```python
from build123d import *

# Parameters (mm, degrees)
F0_W     = 5
F0_H     = 3
F0_W_2   = 14
F3_SIZE  = 0.5
F4_D     = 4.4
F4_DEPTH = 14
F4_TIP   = 1.3218933619
F5_SIZE  = 0.5
F7_D     = 4.4
F7_DEPTH = 14
F7_TIP   = 1.3218933619
F8_W     = 10
F8_H     = 1.5
F9_DEPTH = 10


with BuildPart() as f1:
    # F0 (on Front) → F1 (revolve)
    with BuildSketch(Plane.XZ):
        Polygon((-30.4, 3), (-30.4, 0), (30.4, 0), (30.4, 3), (30.4, 4), (5, 4), (-5, 4), (-30.4, 4), align=None)
        with Locations((-32.9, 1.5)):
            Rectangle(F0_W, F0_H)
        with Locations((37.4, 1.5)):
            Rectangle(F0_W_2, F0_H)
    revolve(axis=Axis((7.3750944167, 0, 0), (1, 0, 0)))

    # F3
    f3_edges = [f1.edges().sort_by_distance(p)[0] for p in [
        (44.4, 0, -3),
    ]]
    chamfer(f3_edges, length=F3_SIZE)

    # F4
    with Locations(Plane.YZ.offset(44.4)):
        with Locations((0, 0)):
            Hole(F4_D / 2, depth=F4_DEPTH)
            with Locations((0, 0, -(F4_DEPTH + F4_TIP / 2))):  # 118° drill point
                Cone(0, F4_D / 2, F4_TIP, mode=Mode.SUBTRACT)

    # F5
    f5_edges = [f1.edges().sort_by_distance(p)[0] for p in [
        (-35.4, 0, -3),
    ]]
    chamfer(f5_edges, length=F5_SIZE)

    # F7
    with Locations(Plane(origin=(-35.4, 0, 0), x_dir=(0, -1, 0), z_dir=(-1, 0, 0))):
        with Locations((0, 0)):
            Hole(F7_D / 2, depth=F7_DEPTH)
            with Locations((0, 0, -(F7_DEPTH + F7_TIP / 2))):  # 118° drill point
                Cone(0, F7_D / 2, F7_TIP, mode=Mode.SUBTRACT)

    # F8 (on Front) → F9 (cut, symmetric)
    with BuildSketch(Plane.XZ):
        with Locations((0.4, -3.25)):
            Rectangle(F8_W, F8_H)
        with Locations((0.4, 3.25)):
            Rectangle(F8_W, F8_H)
    extrude(amount=F9_DEPTH, both=True, mode=Mode.SUBTRACT)


solid = f1.part
```
CAD build for the part. Positions are in the model's coordinates, mm. A direction names the side the tool comes from. Round coordinates to 2 decimals unless told otherwise and drop trailing zeros. Order: outer loops, then holes, each group sorted by start corner. A loop starts at its lowest first (then second) coordinate and runs counter-clockwise, first axis right, second up. Notation, with made-up numbers: (62, 5) - (79, 5) arc R17 ccw to (79, 9) - close; hole circle Ø6 at (-12.5, 58.5). An arc over 180 degrees is marked (long way). Answer in a Markdown table with one row per item. Add a question column.
(1) 3-axis set-ups, long thin cutter, end or side, ignore diameter. For faces 4 (the face through (-4.6, 0, -3)), 5 (the face through (-0.426, 3.549, 1.846)), 6 (the face through (-33, 0, -3)), 7 (the face through (5.4, 0, 3)), 8 (the face through (37.3, -2.1, 0.66)): which of +Z, -Z, +X, -X, +Y, -Y reach the whole face in a straight line?
(2) Band-saw the part on A-A on x = 38. List the corners of the cut face in (y, z).
(3) Probe L1, parallel to Y at x = 41.75, z = 0; L2, parallel to Y at x = -26, z = 0. List the from-to ranges inside material, lowest first. Write a range as [from, to].
(4) Band-saw the part on B-B on x = 19.5. List the corners of the cut face in (y, z).
(5) Drop flat-ended pins along their axis: pin 1 Ø4 at (x, y) = (26, 0.5) entering from +Z; pin 2 Ø1 at (x, y) = (33.5, -0.5) entering from -Z; pin 3 Ø3 at (x, y) = (-2, 0) entering from -Z; pin 4 Ø1.5 at (x, y) = (10.5, -2) entering from -Z. Give the stop position or say it passes through.
(6) Mould opens along X. For faces 1 (the face through (-30.4, -3, 1)), 2 (the face through (5.4, 0, -3)), 3 (the face through (-28.3, 2.1, 0.66)) say: +X half, -X half, draft (parallel to the pull), parting line (faces both ways), or undercut.
(7) Band-saw the part on C-C on x = 3. List the corners of the cut face in (y, z), and give its area (3 significant figures).
Data:
| question | item | result |
|---|---|---|
| 1 | face 4 | -Z, +Y, -Y |
| 1 | face 5 | +X, -X |
| 1 | face 6 | -X |
| 1 | face 7 | +Z, +Y, -Y |
| 1 | face 8 | +X |
| 2 | outline | circle Ø6 at (0, 0); hole circle Ø4.4 at (0, 0) |
| 3 | L1 | y = [-3, -2.2], [2.2, 3] |
| 3 | L2 | y = [-4, -2.2], [2.2, 4] |
| 4 | outline | circle Ø8 at (0, 0) |
| 5 | pin 1 | stops at z = 4 |
| 5 | pin 2 | stops at z = -3 |
| 5 | pin 3 | stops at z = -2.5 |
| 5 | pin 4 | stops at z = -3.8 |
| 6 | face 1 | -X half |
| 6 | face 2 | undercut |
| 6 | face 3 | draft |
| 7 | outline | (-3.12, -2.5) - (3.12, -2.5) arc R4 ccw to (3.12, 2.5) - (-3.12, 2.5) arc R4 ccw to start |
| 7 | area | 37.2 mm^2 |
